Solid Edge part; units mm, degrees
sketch "Sketch1" plane through (0, 0, 0) normal (0, -1, 0) x (1, 0, 0)
  line L0 (4.25, 5) -> (4.25, 0)
  line L1 (4.25, 0) -> (2.85, 0)
  line L2 (2.85, 0) -> (2.5, -0.6062)
  line L3 (2.5, -0.6062) -> (2.5, -10)
  line L4 (2.5, -10) -> (0, -10)
  line L5 (2.3, 2.5) -> (0, 1.1721)
  line L6 (2.3, 5) -> (2.3, 2.5)
  line L7 (4.25, 5) -> (2.3, 5)
revolve "RevolvedProtrusion1" add sketch "Sketch1" angle 360 about axis through (0, 0, -6) along (0, 0, 1)
cosmetic_thread "Thread1"
chamfer "chamfer" distance 0.25 angle 45 1 edges at (-2.5, 0, -10)
fillet "head_roundings" radius 0.3 2 edges at (-4.25, 0, 0) (-4.25, 0, 5)
sketch "Sketch2" plane through (0, 0, 5) normal (0, 0, 1) x (0, 1, 0)
  line L0 (-2.3, 1.3279) -> (-2.3, -1.3279)
  line L1 (0, -2.6558) -> (-2.3, -1.3279)
  line L2 (2.3, -1.3279) -> (0, -2.6558)
  line L3 (2.3, 1.3279) -> (2.3, -1.3279)
  line L4 (0, 2.6558) -> (2.3, 1.3279)
  line L5 (-2.3, 1.3279) -> (0, 2.6558)
extrude "Cutout1" cut sketch "Sketch2" against normal up to vertex (2.5 mm away)
properties part number "STD-DIN912-M5x10" material "Galvanized steel"
Can you work these out from the model? Positions are in its coordinate system, mm. A direction names the side the tool comes from. Give positions to 0.01 mm unless a question says otherwise; leave off trailing zeros. Loops run counter-clockwise (first coordinate to the right, second up) from the corner with the lowest first, then second, coordinate; pieces in that order, holes last. Notation, with made-up numbers: M 30.5,24 L 51.5,24 A8 cw 51.5,37 Z; hole C -21,57 d9. An arc over 180 degrees is marked long. One line per item, written item: value.
1) Imagine slicing it at B-B on z = -4. Write out the boundary of the cut face in (x, y).
Geometry check:
outline: C 0,0 d5
2) Thinking about a two-plate mould opening in X: for faces 4 (the face through (-0.087, -0.39, 1.403)), 5 (the face through (2.285, -3.584, 2.469)), 6 (the face through (0, 0, -10)), which applies, +X half, -X half, draft (parallel to the pull), parting line (faces both ways), or undercut?
Geometry check:
face 4: undercut
face 5: parting line
face 6: draft
3) On a 3-axis mill with a long thin cutter (end or side, diameter ignored), from which of +Z, -Z, +X, -X, +Y, -Y can I reach the whole of each face in a straight line? I mean faces 1 (the face through (-1.65, -1.74, 3.77)), 2 (the face through (2, -2, 5)), 3 (the face through (-0.54, 2.44, -5.24)). Say none if no direction works.
Geometry check:
face 1: +Z
face 2: +Z, +X, -X, +Y, -Y
face 3: -Z
4) I'm going to push flat-ended pins straight in: pin 1 (4 mm diameter, centred on y = 0.5, z = -5.5, fed in from +X); pin 2 (5 mm diameter, centred on x = 1.5, y = -2.5, fed in from -Z); pin 3 (0.9 mm diameter, centred on x = -1, y = 1.5, fed in from +Z); pin 4 (1.5 mm diameter, centred on x = 1, z = -1.5, fed in from +Y). Where does each tip first touch, or does it pass through?
Geometry check:
pin 1: stops at x = 2.5
pin 2: stops at z = -10
pin 3: stops at z = 2.47
pin 4: stops at y = 2.49
5) Please list where these lines run through material, in increasing order: line 1 (X direction, y = -1.5, z = 2.75); line 2 (Z direction, x = 1.75, y = 2.5); line 3 (X direction, y = -2.25, z = 3.75).
Geometry check:
line 1: x = -3.98 to -1.79, 1.79 to 3.98
line 2: z = 0 to 5
line 3: x = -3.61 to -1.36, 1.36 to 3.61
